from build123d import *

# Parameters (mm, degrees)
F1_DEPTH = 12.7
F3_DEPTH = 25.4
F4_R     = 6.35
F5_DEPTH = 25.4
F6_R     = 6.35
F7_DEPTH = 12.7


with BuildPart() as f1:
    # F0 (on Top) → F1 (new body)
    with BuildSketch(Plane.XY):
        with BuildLine():
            ThreePointArc((-98.5095974419, 17.1447865009), (-89.9721430512, 13.1994974474), (-86.4897244217, 4.4630111011))
            ThreePointArc((-86.4897244217, 4.4630111011), (-90.4532380754, -4.7545702694), (-99.8698514014, -8.2187642987))
            Line((-99.8698514014, -8.2187642987), (-99.8698514014, -8.2552134991))
            Line((-99.8698514014, -8.2552134991), (-30.0198514014, -8.2552134991))
            ThreePointArc((-30.0198514014, -8.2552134991), (-42.7198514014, 4.4447865009), (-30.0198514014, 17.1447865009))
            Line((-30.0198514014, 17.1447865009), (-98.5095974419, 17.1447865009))
        make_face()
        with BuildLine():
            ThreePointArc((-17.3198514014, 4.4447865009), (-21.0395952804, 13.425042622), (-30.0198514014, 17.1447865009))
            Line((-30.0198514014, 17.1447865009), (-30.0198514014, -8.2552134991))
            ThreePointArc((-30.0198514014, -8.2552134991), (-21.0395952804, -4.5354696201), (-17.3198514014, 4.4447865009))
        make_face()
        with BuildLine():
            Line((-30.0198514014, -8.2552134991), (-30.0198514014, 17.1447865009))
            ThreePointArc((-30.0198514014, 17.1447865009), (-42.7198514014, 4.4447865009), (-30.0198514014, -8.2552134991))
        make_face()
    extrude(amount=F1_DEPTH)

    # F2 (on face) → F3 (join)
    with BuildSketch(Plane(origin=(0, 0, 0), x_dir=(1, 0, 0), z_dir=(0, 0, -1))):
        with BuildLine():
            ThreePointArc((-99.8698514014, -17.0553149368), (-90.4694861278, -13.6064937824), (-86.4898032129, -4.418275319))
            ThreePointArc((-86.4898032129, -4.418275319), (-90.4694861278, 4.7699431443), (-99.8698514014, 8.2187642987))
            Line((-99.8698514014, 8.2187642987), (-99.8698514014, -17.0553149368))
        make_face()
        with BuildLine():
            Line((-99.8698514014, 8.2187642987), (-99.8698514014, 8.2552134991))
            Line((-99.8698514014, 8.2552134991), (-99.8698514014, 8.3082358629))
            ThreePointArc((-99.8698514014, 8.3082358629), (-111.8897244217, -4.373539537), (-99.8698514014, -17.0553149368))
            Line((-99.8698514014, -17.0553149368), (-99.8698514014, 8.2187642987))
        make_face()
    extrude(amount=-F3_DEPTH)

    # F4 (on face) → F5 (cut)
    with BuildSketch(Plane.XY.offset(25.4)):
        with Locations((-99.1897244217, 4.373539537)):
            Circle(F4_R)
    extrude(amount=-F5_DEPTH, mode=Mode.SUBTRACT)

    # F6 (on face) → F7 (cut)
    with BuildSketch(Plane.XY.offset(12.7)):
        with Locations((-30.0198514014, 4.4447865009)):
            Circle(F6_R)
    extrude(amount=-F7_DEPTH, mode=Mode.SUBTRACT)


solid = f1.part
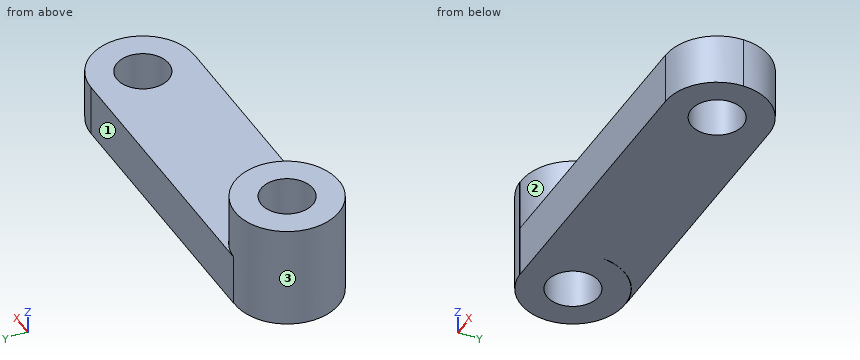
Read the model definition and answer for the solid it produces. Units are mm, in the model's axes. Face numbers are marked on the shaded views. Give positions to 0.01 mm unless a question says otherwise; leave off trailing zeros. Write each loop counter-clockwise with the first axis right and the second up, starting at its lowest first coordinate (ties: lowest second). Pieces come first, ordered by that corner, then holes. Notation, with made-up numbers: (64.25, -11.75) - (83.25, -11.75) arc R25 cw to (83.25, 14.25) - close; hole circle Ø5 at (10, -22). An arc over 180 degrees is marked (long way). Use CSV: the item, a comma, the result in double quotes. Start each with the question number.
(1) Find section C-C (x = -31). Give the vertices of the cut face in (y, z).
(2) Find section B-B (y = 5.5). Give the vertices of the cut face in (x, z), plus the area to 3 significant figures.
(3) Find section D-D (y = 13.25). Give the vertices of the cut face in (x, z).
(4) Consider line 1 along Z through (x, y) = (-32, -5.5); line 2 along Y through (x, z) = (-76.5, 11); line 3 along X through (y, z) = (0.5, 22.25). Determine where each line is inside the solid, lowest interval first.
(5) Find section A-A (y = -0.25). Give the vertices of the cut face in (x, z), plus the area to 3 significant figures.
(6) Determine the mould class of the marked faces 1, 2 and 3 for opening direction Y: +Y half, -Y half, draft (parallel to the pull), parting line (faces both ways), or undercut.
(7) Given P1, Ø2, axis at x = -88, z = 18, coming from the +Y side; P2, Ø5, axis at y = 9, z = 18.5, coming from the -X side; P3, Ø12, axis at y = -2, z = 5.5, coming from the -X side, each flat-ended and moving along its own axis, determine where each tip first touches the part or whether it passes through.
Findings below:
1,outline,"(-8.26, 0) - (-1.83, 0) - (-1.83, 12.7) - (-8.26, 12.7) - close; (10.72, 0) - (17.14, 0) - (17.14, 12.7) - (10.72, 12.7) - close"
2,outline,"(-111.84, 0) - (-105.44, 0) - (-105.44, 25.4) - (-111.84, 25.4) - close; (-92.94, 0) - (-86.54, 0) - (-86.54, 25.4) - (-92.94, 25.4) - close; (-86.53, 0) - (-36.28, 0) - (-36.28, 12.7) - (-86.53, 12.7) - close; (-23.76, 0) - (-17.36, 0) - (-17.36, 12.7) - (-23.76, 12.7) - close"
2,area,"1,040 mm2"
3,outline,"(-108.27, 0) - (-90.11, 0) - (-90.11, 25.4) - (-108.27, 25.4) - close; (-90.02, 0) - (-20.87, 0) - (-20.87, 12.7) - (-90.02, 12.7) - close"
4,line 1,"0 to 12.7"
4,line 2,"-8.26 to 17.14"
4,line 3,"-111.28 to -104.22, -94.16 to -87.12"
5,outline,"(-111.02, 0) - (-103.54, 0) - (-103.54, 25.4) - (-111.02, 25.4) - close; (-94.84, 0) - (-34.3, 0) - (-34.3, 12.7) - (-87.4, 12.7) - (-87.4, 25.4) - (-94.84, 25.4) - close; (-25.74, 0) - (-18.22, 0) - (-18.22, 12.7) - (-25.74, 12.7) - close"
5,area,"1,150 mm2"
6,face 1,"+Y half"
6,face 2,"-Y half"
6,face 3,"undercut"
7,P1,"y = 11.95"
7,P2,"x = -111.71"
7,P3,"x = -111.88"
